```python
from build123d import *

# Parameters (mm, degrees)
SKETCH1_R           = 5.5
BOSS_EXTRUDE1_DEPTH = 75
BOSS_EXTRUDE2_DEPTH = 22
SKETCH3_R           = 2
CUT_EXTRUDE1_DEPTH  = 100.249870156
SKETCH4_W           = 3
SKETCH4_H           = 12
CUT_EXTRUDE2_DEPTH  = 13
SKETCH5_R           = 4
BOSS_EXTRUDE3_DEPTH = 10
BOSS_EXTRUDE4_START = 13
BOSS_EXTRUDE4_DEPTH = 13
SKETCH7_R           = 3.5
BOSS_EXTRUDE5_DEPTH = 10
SKETCH9_R           = 4
BOSS_EXTRUDE6_DEPTH = 8
SKETCH10_R          = 2
CUT_EXTRUDE3_DEPTH  = 80


with BuildPart() as part:
    # Sketch1 → Boss-Extrude1 (new body)
    with BuildSketch(Plane(origin=(0, 0, 0), x_dir=(1, 0, 0), z_dir=(0, 1, 0))):
        with Locations(Location((-60.059570612, 11.249252908, 0), (0, 0, 270))):
            Circle(SKETCH1_R)
    extrude(amount=BOSS_EXTRUDE1_DEPTH)

    # Sketch2 → Boss-Extrude2 (add)
    with BuildSketch(Plane(origin=(0, 75, 0), x_dir=(1, 0, 0), z_dir=(0, 1, 0))):
        with BuildLine():
            Line((-63.059570612, 17.249252908), (-57.059570612, 17.249252908))
            ThreePointArc((-57.059570612, 17.249252908), (-54.938250268, 16.370573252), (-54.059570612, 14.249252908))
            Line((-54.059570612, 14.249252908), (-54.059570612, 8.249252908))
            ThreePointArc((-54.059570612, 8.249252908), (-54.938250268, 6.127932565), (-57.059570612, 5.249252908))
            Line((-57.059570612, 5.249252908), (-63.059570612, 5.249252908))
            ThreePointArc((-63.059570612, 5.249252908), (-65.180890956, 6.127932565), (-66.059570612, 8.249252908))
            Line((-66.059570612, 8.249252908), (-66.059570612, 14.249252908))
            ThreePointArc((-66.059570612, 14.249252908), (-65.180890956, 16.370573252), (-63.059570612, 17.249252908))
        make_face()
    extrude(amount=BOSS_EXTRUDE2_DEPTH)

    # Sketch3 → Cut-Extrude1 (cut, through all)
    with BuildSketch(Plane.ZY.offset(66.059570612)):
        with Locations((-11.249252908, 92)):
            Circle(SKETCH3_R)
    extrude(amount=-CUT_EXTRUDE1_DEPTH, mode=Mode.SUBTRACT)

    # Sketch4 → Cut-Extrude2 (cut)
    with BuildSketch(Plane(origin=(0, 97, 0), x_dir=(1, 0, 0), z_dir=(0, 1, 0))):
        with Locations((-60.059570612, 11.249252908)):
            Rectangle(SKETCH4_W, SKETCH4_H)
    extrude(amount=-CUT_EXTRUDE2_DEPTH, mode=Mode.SUBTRACT)

    # Sketch5 → Boss-Extrude3 (add)
    with BuildSketch(Plane(origin=(0, 0, -17.249252908), x_dir=(-1, 0, 0), z_dir=(0, 0, -1))):
        with Locations(Location((60.059570612, 79.5, 0), (0, 0, 138.590377891))):
            Circle(SKETCH5_R)
    extrude(amount=BOSS_EXTRUDE3_DEPTH)

    # Sketch6 → Boss-Extrude4 (add)
    with BuildSketch(Plane.XZ.offset(BOSS_EXTRUDE4_START)):
        with BuildLine():
            Line((-57.059570612, -17.249252908), (-63.059570612, -17.249252908))
            ThreePointArc((-63.059570612, -17.249252908), (-65.180890956, -16.370573252), (-66.059570612, -14.249252908))
            Line((-66.059570612, -14.249252908), (-66.059570612, -8.249252908))
            ThreePointArc((-66.059570612, -8.249252908), (-65.180890956, -6.127932565), (-63.059570612, -5.249252908))
            Line((-63.059570612, -5.249252908), (-57.059570612, -5.249252908))
            ThreePointArc((-57.059570612, -5.249252908), (-54.938250268, -6.127932565), (-54.059570612, -8.249252908))
            Line((-54.059570612, -8.249252908), (-54.059570612, -14.249252908))
            ThreePointArc((-54.059570612, -14.249252908), (-54.938250268, -16.370573252), (-57.059570612, -17.249252908))
        make_face()
    extrude(amount=-BOSS_EXTRUDE4_DEPTH)

    # Sketch7 → Boss-Extrude5 (add)
    with BuildSketch(Plane(origin=(0, 0, -17.249252908), x_dir=(-1, 0, 0), z_dir=(0, 0, -1))):
        with Locations(Location((60.059570612, -4.5, 0), (0, 0, 148.997280866))):
            Circle(SKETCH7_R)
    extrude(amount=BOSS_EXTRUDE5_DEPTH)

    # Sketch9 → Boss-Extrude6 (add)
    with BuildSketch(Plane.XZ.offset(13)):
        with Locations(Location((-60.059570612, -11.249252908, 0), (0, 0, 90))):
            Circle(SKETCH9_R)
    extrude(amount=BOSS_EXTRUDE6_DEPTH)

    # Sketch10 → Cut-Extrude3 (cut)
    with BuildSketch(Plane.XZ.offset(21)):
        with Locations(Location((-60.059570612, -11.249252908, 0), (0, 0, 270))):
            Circle(SKETCH10_R)
    extrude(amount=-CUT_EXTRUDE3_DEPTH, mode=Mode.SUBTRACT)


solid = part.part
```
Here's how the part is built. I have some questions about the finished solid (model axes, mm). A direction names the side the tool comes from. Coordinates: 2 decimals unless noted, no trailing zeros. Write each loop counter-clockwise with the first axis right and the second up, starting at its lowest first coordinate (ties: lowest second). Pieces come first, ordered by that corner, then holes. Notation, with made-up numbers: (31.5, -16.75) -> (57.5, -16.75) arc R30 ccw to (57.5, 19.25) -> close; hole circle Ø5 at (75.25, 48). An arc over 180 degrees is marked (long way). Use a Markdown table: item, result. Add a question column.
(1) We'd pull the mould along Z, two halves only. Please class faces 5 (the cylindrical face through (-65.2, -6.59, -6.15)), 6 (the cylindrical face through (-65.43, 36.98, -12.44)), 7 (the cylindrical face through (-63.841, 93.983, -11.51)), 8 (the cylindrical face through (-62.47, -1.96, -22.18)): +Z half, -Z half, draft (parallel to the pull), parting line (faces both ways), or undercut.
(2) If we section it at C-C, the plane z = -23: Write out the boundary of the cut face in (x, y).
(3) If we section it at B-B, the plane y = -4.5: Write out the boundary of the cut face in (x, z), and give its area (3 significant figures).
(4) Please list where these lines run through material, in increasing order: line 1 (Y direction, x = -62.5, z = -11); line 2 (Y direction, x = -60.5, z = -8.5); line 3 (X direction, y = 3.5, z = -11.5).
(5) I'm going to push flat-ended pins straight in: P1, Ø2.5, axis at x = -60.06, z = -11.25, coming from the +Y side; P2, Ø3, axis at x = -63.5, y = 41.5, coming from the -Z side; P3, Ø5, axis at x = -56, y = 43.5, coming from the -Z side. Where does each tip first touch, or does it pass through?
(6) If we section it at A-A, the plane y = 92: Write out the boundary of the cut face in (x, z), and give its area (3 significant figures).
(7) If we section it at D-D, the plane y = 79.5: Write out the boundary of the cut face in (x, z).
(8) For faces 1 (the flat face through (-60, 84, -11)), 2 (the cylindrical face through (-58.3, 83.09, -22.18)), 3 (the flat face through (-63, 0, -6)), 4 (the flat face through (-62, -21, -10)), which set-ups out of +Z, -Z, +X, -X, +Y, -Y let a thin tool reach every point of the face, with its end or its side?
Outcome:
| question | item | result |
|---|---|---|
| 1 | face 5 | +Z half |
| 1 | face 6 | parting line |
| 1 | face 7 | undercut |
| 1 | face 8 | draft |
| 2 | outline | circle Ø8 at (-60.06, 79.5); circle Ø7 at (-60.06, -4.5) |
| 3 | outline | (-66.06, -14.25) arc R3 ccw to (-63.06, -17.25) -> (-63.56, -17.25) -> (-63.56, -27.25) -> (-56.56, -27.25) -> (-56.56, -17.25) -> (-57.06, -17.25) arc R3 ccw to (-54.06, -14.25) -> (-54.06, -8.25) arc R3 ccw to (-57.06, -5.25) -> (-63.06, -5.25) arc R3 ccw to (-66.06, -8.25) -> close; hole circle Ø4 at (-60.06, -11.25) |
| 3 | area | 194 mm^2 |
| 4 | line 1 | y = -21 to 90.02, 93.98 to 97 |
| 4 | line 2 | y = -21 to 84 |
| 4 | line 3 | x = -65.55 to -62.04, -58.08 to -54.57 |
| 5 | P1 | stops at y = 84 |
| 5 | P2 | stops at z = -16.4 |
| 5 | P3 | stops at z = -16.52 |
| 6 | outline | (-66.06, -14.25) arc R3 ccw to (-63.06, -17.25) -> (-61.56, -17.25) -> (-61.56, -13.25) -> (-66.06, -13.25) -> close; (-66.06, -9.25) -> (-61.56, -9.25) -> (-61.56, -5.25) -> (-63.06, -5.25) arc R3 ccw to (-66.06, -8.25) -> close; (-58.56, -17.25) -> (-57.06, -17.25) arc R3 ccw to (-54.06, -14.25) -> (-54.06, -13.25) -> (-58.56, -13.25) -> close; (-58.56, -9.25) -> (-54.06, -9.25) -> (-54.06, -8.25) arc R3 ccw to (-57.06, -5.25) -> (-58.56, -5.25) -> close |
| 6 | area | 64.3 mm^2 |
| 7 | outline | (-66.06, -14.25) arc R3 ccw to (-63.06, -17.25) -> (-64.06, -17.25) -> (-64.06, -27.25) -> (-56.06, -27.25) -> (-56.06, -17.25) -> (-57.06, -17.25) arc R3 ccw to (-54.06, -14.25) -> (-54.06, -8.25) arc R3 ccw to (-57.06, -5.25) -> (-63.06, -5.25) arc R3 ccw to (-66.06, -8.25) -> close |
| 8 | face 1 | +Z, -Z, +Y |
| 8 | face 2 | -Z |
| 8 | face 3 | none |
| 8 | face 4 | +Z, -Z, +X, -X, -Y |
